Source: CAD feature listing. Evaluate the final solid. Frame: model axes, mm. Face numbers are marked on the shaded views. A direction names the side the tool comes from. Give positions to 0.01 mm unless a question says otherwise; leave off trailing zeros. Write each loop counter-clockwise with the first axis right and the second up, starting at its lowest first coordinate (ties: lowest second). Pieces come first, ordered by that corner, then holes. Notation, with made-up numbers: M 38.25,35 L 82.25,35 A29 cw 82.25,68 Z; hole C 39,-10 d7. An arc over 180 degrees is marked long. Use CSV: the item, a comma, the result in double quotes. Start each with the question number.
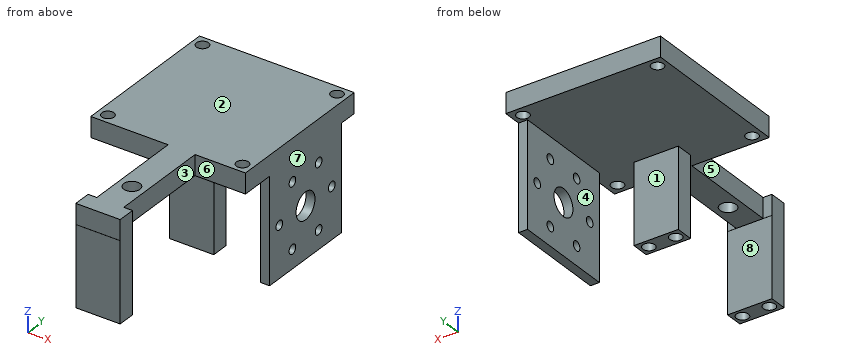
from build123d import *

# Parameters (mm, degrees)
SKETCH014_R             = 3
SKETCH014_R_2           = 2.25
PAD007_DEPTH            = 7.5
SKETCH015_W             = 16.5
SKETCH015_H             = 6.5
SKETCH015_R             = 2.25
PAD008_DEPTH            = 29.65
PAD010_DEPTH            = 39
SKETCH017_R             = 5
SKETCH017_R_2           = 1.75
POCKET_DEPTH            = 5
BODY002_PLACEMENT_ANGLE = 180


with BuildPart() as part:
    # Sketch014 → Pad007 (new body)
    with BuildSketch(Plane.XY):
        Polygon((0, -28.75), (0, -55), (0, -66.44), (3.25, -66.44), (3.25, -72.94), (-13.25, -72.94), (-13.25, -66.44), (-10, -66.44), (-10, -55), (-10, -28.75), (-28.75, -28.75), (-28.75, 28.75), (28.75, 28.75), (28.75, -28.75), align=None)
        with Locations((-5, -55)):
            Circle(SKETCH014_R, mode=Mode.SUBTRACT)
        with Locations((-25, -25)):
            Circle(SKETCH014_R_2, mode=Mode.SUBTRACT)
        with Locations((25, 25)):
            Circle(SKETCH014_R_2, mode=Mode.SUBTRACT)
        with Locations((25, -25)):
            Circle(SKETCH014_R_2, mode=Mode.SUBTRACT)
        with Locations((-25, 25)):
            Circle(SKETCH014_R_2, mode=Mode.SUBTRACT)
    extrude(amount=PAD007_DEPTH)

    # Sketch015 (on Face21 of Pad007) → Pad008 (join)
    with BuildSketch(Plane.XY.offset(7.5)):
        with Locations((-5, -20.21)):
            Rectangle(SKETCH015_W, SKETCH015_H)
        with Locations((-10, -20.21)):
            Circle(SKETCH015_R, mode=Mode.SUBTRACT)
        with Locations((0, -20.21)):
            Circle(SKETCH015_R, mode=Mode.SUBTRACT)
        with Locations((-5, -69.71)):
            Rectangle(SKETCH015_W, SKETCH015_H)
        with Locations((0, -69.71)):
            Circle(SKETCH015_R, mode=Mode.SUBTRACT)
        with Locations((-10, -69.71)):
            Circle(SKETCH015_R, mode=Mode.SUBTRACT)
    extrude(amount=PAD008_DEPTH)

    # Sketch016 (on Face5 of Pad008) → Pad010 (join)
    with BuildSketch(Plane.XY.offset(7.5)):
        Polygon((-25.4, 3), (-25.4, 22), (-28.75, 22), (-28.75, -16), (-25.4, -16), align=None)
    extrude(amount=PAD010_DEPTH)

    # Sketch017 (on Face7 of Pad010) → Pocket (cut)
    with BuildSketch(Plane(origin=(-28.75, 0, 0), x_dir=(0, -1, 0), z_dir=(-1, 0, 0))):
        with Locations((-3, 27.5)):
            Circle(SKETCH017_R)
        with Locations((3.93, 39.5)):
            Circle(SKETCH017_R_2)
        with Locations((-9.93, 39.5)):
            Circle(SKETCH017_R_2)
        with Locations((-9.93, 15.5)):
            Circle(SKETCH017_R_2)
        with Locations((3.93, 15.5)):
            Circle(SKETCH017_R_2)
        with Locations((-16.865388, 27.5)):
            Circle(SKETCH017_R_2)
        with Locations((10.865388, 27.5)):
            Circle(SKETCH017_R_2)
    extrude(amount=-POCKET_DEPTH, mode=Mode.SUBTRACT)


with BuildPart() as part_1:
    # Body002 placement: moved
    add(part.part.rotate(Axis((0, 0, 0), (0, 1, 0)), BODY002_PLACEMENT_ANGLE))


solid = part_1.part
1. Line query: probe 1 along X at (y, z) = (-20, -25); probe 2 along Z at (x, y) = (28.05, 9.93); probe 3 along Y at (x, z) = (-25, -3.75). Output: solid intervals per line, ascending.
2. Section B-B on y = 3. Return loops of the section in (x, z).
3. First-contact query: pin 1 (2 mm diameter, centred on x = 10, y = -19, fed in from -Z); pin 2 (1.7 mm diameter, centred on x = 27.5, z = -28, fed in from -Y); pin 3 (8.5 mm diameter, centred on x = 8, z = -23, fed in from +Y); pin 4 (2 mm diameter, centred on y = 9.5, z = -14, fed in from +X). Flat tips, straight axial feed; report the tip coordinate or a pass-through.
4. Section D-D on z = -27.5. Give the number of separate pieces and of enclosed holes in the cut face, then the cut area to 3 significant figures.
5. Section A-A on z = -10.5. Return loops of the section in (x, y), then the cut area to 3 significant figures.
6. Section C-C on x = -25. Return loops of the section in (y, z).
7. Pull-direction query (Y, two-part tool) for the marked faces 1, 2 and 3; classes: released by +Y, released by -Y, zero draft, split by the parting line, or undercut.
8. Access query for the marked faces 4, 5, 6, 7 and 8. Directions: +Z, -Z, +X, -X, +Y, -Y. A direction counts if a zero-diameter tool reaches every point of the face in a straight line with its end or side. Return the directions, or none.
Resolved:
1,probe 1,"x = -3.25 to -2.24, 2.24 to 7.76, 12.24 to 13.25"
1,probe 2,"z = -46.5 to -41.25, -37.75 to -17.25, -13.75 to 0"
1,probe 3,"y = -28.75 to -27.25, -22.75 to 22.75, 27.25 to 28.75"
2,outline,"M -28.75,-7.5 L 25.4,-7.5 L 25.4,-22.5 L 28.75,-22.5 L 28.75,0 L -28.75,0 Z; M 25.4,-46.5 L 28.75,-46.5 L 28.75,-32.5 L 25.4,-32.5 Z"
3,pin 1,"stops at z = -7.5"
3,pin 2,"stops at y = -16"
3,pin 3,"stops at y = -16.96"
3,pin 4,"stops at x = 28.75"
4,separate pieces,"6"
4,enclosed holes,"4"
4,area,"221 mm2"
5,outline,"M -3.25,-72.96 L 13.25,-72.96 L 13.25,-66.46 L -3.25,-66.46 Z; M -3.25,-23.46 L 13.25,-23.46 L 13.25,-16.96 L -3.25,-16.96 Z; M 25.4,-16 L 28.75,-16 L 28.75,22 L 25.4,22 Z; hole C 0,-69.71 d4.5; hole C 0,-20.21 d4.5; hole C 10,-69.71 d4.5; hole C 10,-20.21 d4.5"
5,area,"278 mm2"
6,outline,"M -28.75,-7.5 L -27.25,-7.5 L -27.25,0 L -28.75,0 Z; M -22.75,-7.5 L 22.75,-7.5 L 22.75,0 L -22.75,0 Z; M 27.25,-7.5 L 28.75,-7.5 L 28.75,0 L 27.25,0 Z"
7,face 1,"released by +Y"
7,face 2,"zero draft"
7,face 3,"undercut"
8,face 4,"-Z, -X, +Y, -Y"
8,face 5,"+Z, -Z, -X"
8,face 6,"+Z, -Z, +X"
8,face 7,"+Z, -Z, +X, +Y, -Y"
8,face 8,"-Z, +X, -X"
